from build123d import *

# Parameters (mm, degrees)
SKETCH_1_W          = 5
SKETCH_1_H          = 7
EXTRUDE_2_DEPTH     = 140
FILLET_1_R          = 3.5
SKETCH_3_R          = 1.55
CUT_EXTRUDE_1_DEPTH = 141.132972565
SKETCH_4_W          = 2.5
SKETCH_4_H          = 7
EXTRUDE_3_DEPTH     = 7
FILLET_2_R          = 3.5
SKETCH_5_R          = 1.55
CUT_EXTRUDE_2_DEPTH = 148.062911708


with BuildPart() as part:
    # 草图1 → 凸台-拉伸2 (new body)
    with BuildSketch(Plane.XY):
        Rectangle(SKETCH_1_W, SKETCH_1_H)
    extrude(amount=EXTRUDE_2_DEPTH)

    # 圆角1
    fillet_1_edges = [part.edges().sort_by_distance(p)[0] for p in [
        (0, -3.5, 0),
        (0, 3.5, 0),
    ]]
    fillet(fillet_1_edges, radius=FILLET_1_R - 0.0001)  # a hair under: the kernel refuses the full size

    # 草图3 → 切除-拉伸1 (cut, through all)
    with BuildSketch(Plane(origin=(2.5, 0, 0), x_dir=(0, 0, -1), z_dir=(1, 0, 0))):
        with Locations(Location((-3.5, 0, 0), (0, 0, 90))):
            Circle(SKETCH_3_R)
    extrude(amount=-CUT_EXTRUDE_1_DEPTH, mode=Mode.SUBTRACT)

    # 草图4 → 凸台-拉伸3 (add)
    with BuildSketch(Plane.XY.offset(140)):
        with Locations((1.25, 0)):
            Rectangle(SKETCH_4_W, SKETCH_4_H)
    extrude(amount=EXTRUDE_3_DEPTH)

    # 圆角2
    fillet_2_edges = [part.edges().sort_by_distance(p)[0] for p in [
        (1.25, -3.5, 147),
        (1.25, 3.5, 147),
    ]]
    fillet(fillet_2_edges, radius=FILLET_2_R - 0.0001)  # a hair under: the kernel refuses the full size

    # 草图5 → 切除-拉伸2 (cut, through all)
    with BuildSketch(Plane.ZY):
        with Locations(Location((143.5, 0, 0), (0, 0, 270))):
            Circle(SKETCH_5_R)
    extrude(amount=-CUT_EXTRUDE_2_DEPTH, mode=Mode.SUBTRACT)


solid = part.part
Can you work these out from the model? Positions are in its coordinate system, mm. A direction names the side the tool comes from. Coordinates: 2 decimals unless noted, no trailing zeros. Return JSON: item names as keys, results as strings. Group by question number.
Item 1: If I drill on L1, parallel to Z at x = 0.35, y = 0; L2, parallel to Z at x = -0.4, y = 0; L3, parallel to Y at x = 1.6, z = 143.5, over which ranges is the centre line in solid material (lowest first)? Write a range as from..to.
Item 2: I'm going to push a flat-ended pin straight in: pin 1 Ø1.9 at (y, z) = (0, 143.5) entering from +X. Where does the tip first touch, or does it pass through?
Item 3: On a 3-axis mill with a long thin cutter (end or side, diameter ignored), from which of +Z, -Z, +X, -X, +Y, -Y can I reach the whole of each face in a straight line? I mean faces 5 (the flat face through (-2.5, 0, 69)), 6 (the flat face through (-1, 0, 140)). Say none if no direction works.
Item 4: Thinking about a two-plate mould opening in Z: for faces 1 (the cylindrical face through (0.04, 2.5, 1.05)), 2 (the flat face through (2.5, 0, 72)), 3 (the cylindrical face through (0.035, -0.202, 5.037)), 4 (the cylindrical face through (1.27, -2.45, 146)), which applies, released by +Z, released by -Z, zero draft, split by the parting line, or undercut?
Item 5: Imagine slicing it at A-A (x = 1). Give the number of separate pieces and of enclosed holes in the cut face, and give its area (3 significant figures).
Verdict:
{
 "1": {"L1": "z = 0..1.95, 5.05..141.95, 145.05..147", "L2": "z = 0..1.95, 5.05..140", "L3": "y = -3.5..-1.55, 1.55..3.5"},
 "2": {"pin 1": "passes through"},
 "3": {"face 5": "+Z, -Z, -X, +Y, -Y", "face 6": "+Z, -X, +Y, -Y"},
 "4": {"face 1": "released by -Z", "face 2": "zero draft", "face 3": "undercut", "face 4": "released by +Z"},
 "5": {"separate pieces": "1", "enclosed holes": "2", "area": "1,000 mm^2"}
}
